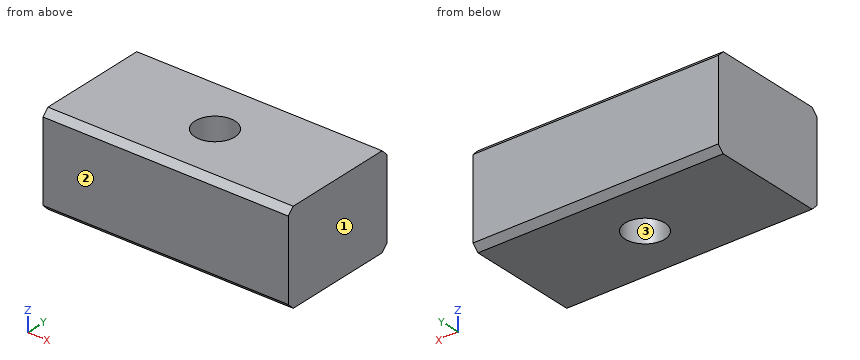
from build123d import *

# Parameters (mm, degrees)
F0_W     = 40
F0_H     = 20
F1_DEPTH = 15
F3_D     = 6.5
F4_SIZE  = 1
F5_SIZE  = 1


with BuildPart() as f1:
    # F0 (on Top) → F1 (new body)
    with BuildSketch(Plane.XY):
        with Locations((20, 10)):
            Rectangle(F0_W, F0_H)
    extrude(amount=F1_DEPTH)

    # F3 (through all)
    with Locations(Plane.XY.offset(15)):
        with Locations((20, 10)):
            Hole(F3_D / 2)

    # F4
    f4_edges = [f1.edges().sort_by_distance(p)[0] for p in [
        (20, 0, 15),
        (20, 20, 15),
    ]]
    chamfer(f4_edges, length=F4_SIZE)

    # F5
    f5_edges = [f1.edges().sort_by_distance(p)[0] for p in [
        (20, 0, 0),
        (20, 20, 0),
    ]]
    chamfer(f5_edges, length=F5_SIZE)


solid = f1.part
The listing builds one solid part. Answer for the finished solid, in the listing's coordinates (mm). Face numbers are marked on the shaded views. Give positions to 0.01 mm unless a question says otherwise; leave off trailing zeros. Order: outer loops, then holes, each group sorted by start corner. A loop starts at its lowest first (then second) coordinate and runs counter-clockwise, first axis right, second up. Notation, with made-up numbers: (83, 72.25) -> (97, 72.25) arc R21 ccw to (97, 99.25) -> close; hole circle Ø10 at (-7, 9). An arc over 180 degrees is marked (long way). Put each result on its own line as item: value.
Item 1: For a pull along Y with two mould halves and no side action, classify the marked faces 1, 2 and 3 as released by +Y, released by -Y, zero draft, split by the parting line, or undercut.
Established:
face 1: zero draft
face 2: released by -Y
face 3: undercut
Item 2: A cutting plane is placed at D-D on y = 8. Give the vertices of the cut face in (x, z), plus the area to 3 significant figures.
Established:
outline: (0, 0) -> (17.44, 0) -> (17.44, 15) -> (0, 15) -> close; (22.56, 0) -> (40, 0) -> (40, 15) -> (22.56, 15) -> close
area: 523 mm^2
Item 3: A cutting plane is placed at B-B on x = 20. Give the vertices of the cut face in (y, z).
Established:
outline: (0, 1) -> (1, 0) -> (6.75, 0) -> (6.75, 15) -> (1, 15) -> (0, 14) -> close; (13.25, 0) -> (19, 0) -> (20, 1) -> (20, 14) -> (19, 15) -> (13.25, 15) -> close
Item 4: Straight lines are drawn through the part: line 1 (Y direction, x = 20, z = 9.5); line 2 (X direction, y = 7.25, z = 9.75); line 3 (X direction, y = 11.5, z = 2). For each, find the intervals that lie inside material, in ascending order.
Established:
line 1: y = 0 to 6.75, 13.25 to 20
line 2: x = 0 to 18.27, 21.73 to 40
line 3: x = 0 to 17.12, 22.88 to 40
Item 5: A cutting plane is placed at A-A on y = 10. Give the vertices of the cut face in (x, z).
Established:
outline: (0, 0) -> (16.75, 0) -> (16.75, 15) -> (0, 15) -> close; (23.25, 0) -> (40, 0) -> (40, 15) -> (23.25, 15) -> close
Item 6: A cutting plane is placed at C-C on z = 5.75. Give the vertices of the cut face in (x, y), plus the area to 3 significant figures.
Established:
outline: (0, 0) -> (40, 0) -> (40, 20) -> (0, 20) -> close; hole circle Ø6.5 at (20, 10)
area: 767 mm^2
Item 7: Given P1, Ø6, axis at x = 20, y = 10, coming from the +Z side, flat-ended and moving along its own axis, determine where the tip first touches the part or whether it passes through.
Established:
P1: passes through
